```python
from build123d import *

# Parameters (mm, degrees)
SKETCH1_R               = 10
SKETCH1_R_2             = 4.425
BOSS_EXTRUDE1_DEPTH     = 2
SKETCH1_2_R             = 4.425
BOSS_EXTRUDE2_DEPTH     = 4.55
SKETCH2_R               = 2.75
SKETCH2_R_2             = 1.5
CUT_EXTRUDE1_DEPTH      = 3.5
CUT_EXTRUDE2_DEPTH      = 15.85605937
CUT_EXTRUDE2_DEPTH_BACK = 15.85605937
SKETCH2_3_R             = 1.5
SKETCH3_R               = 1.5
CUT_EXTRUDE3_DEPTH      = 15.370194849
CIRPATTERN1_COUNT       = 4
FILLET1_R               = 0.5


with BuildPart() as part:
    # Sketch1 → Boss-Extrude1 (new body)
    with BuildSketch(Plane(origin=(0, 0, 0), x_dir=(1, 0, 0), z_dir=(0, 1, 0))):
        with Locations(Location((0, 0, 0), (0, 0, 270))):
            Circle(SKETCH1_R)
        with Locations(Location((0, 0, 0), (0, 0, 270))):
            Circle(SKETCH1_R_2, mode=Mode.SUBTRACT)
    extrude(amount=BOSS_EXTRUDE1_DEPTH)

    # Sketch1_2 → Boss-Extrude2 (add)
    with BuildSketch(Plane(origin=(0, 0, 0), x_dir=(1, 0, 0), z_dir=(0, 1, 0))):
        with Locations(Location((0, 0, 0), (0, 0, 270))):
            Circle(SKETCH1_2_R)
    extrude(amount=BOSS_EXTRUDE2_DEPTH)

    # Sketch2 → Cut-Extrude1 (cut)
    # profile 1 of 2: a face of its own
    with BuildSketch(Plane(origin=(0, 4.55, 0), x_dir=(1, 0, 0), z_dir=(0, 1, 0))):
        with Locations(Location((0, 0, 0), (0, 0, 270))):
            Circle(SKETCH2_R)
        Circle(SKETCH2_R_2, mode=Mode.SUBTRACT)
    # profile 2 of 2: a face of its own
    with BuildSketch(Plane(origin=(0, 4.55, 0), x_dir=(1, 0, 0), z_dir=(0, 1, 0))):
        Circle(SKETCH2_R_2)
    extrude(amount=-CUT_EXTRUDE1_DEPTH, mode=Mode.SUBTRACT)

    # Sketch2_3 → Cut-Extrude2 (cut, two sides: drawn at the far end of the back side and taken through both)
    with BuildSketch(Plane(origin=(0, 4.55, 0), x_dir=(1, 0, 0), z_dir=(0, 1, 0)).offset(-CUT_EXTRUDE2_DEPTH_BACK)):
        with Locations(Location((0, 0, 0), (0, 0, 270))):
            Circle(SKETCH2_3_R)
    extrude(amount=CUT_EXTRUDE2_DEPTH + CUT_EXTRUDE2_DEPTH_BACK, mode=Mode.SUBTRACT)

    # Sketch3 → Cut-Extrude3 (cut, symmetric)
    with BuildSketch(Plane(origin=(0, 2, 0), x_dir=(1, 0, 0), z_dir=(0, 1, 0))):
        with Locations(Location((0, 7.2125, 0), (0, 0, 270))):
            Circle(SKETCH3_R)
    cut_extrude3 = extrude(amount=CUT_EXTRUDE3_DEPTH, both=True, mode=Mode.SUBTRACT)

    # CirPattern1: Cut-Extrude3 ×4 about axis
    cirpattern1_axis = Axis((0, 0, 0), (0, 1, 0))
    for i in range(1, CIRPATTERN1_COUNT):
        add(cut_extrude3.rotate(cirpattern1_axis, i * 360 / CIRPATTERN1_COUNT), mode=Mode.SUBTRACT)

    # Fillet1
    fillet1_edges = [part.edges().sort_by_distance(p)[0] for p in [
        (0, 4.55, -4.425),
        (0, 0, -10),
        (0, 2, -10),
    ]]
    fillet(fillet1_edges, radius=FILLET1_R)


solid = part.part
```
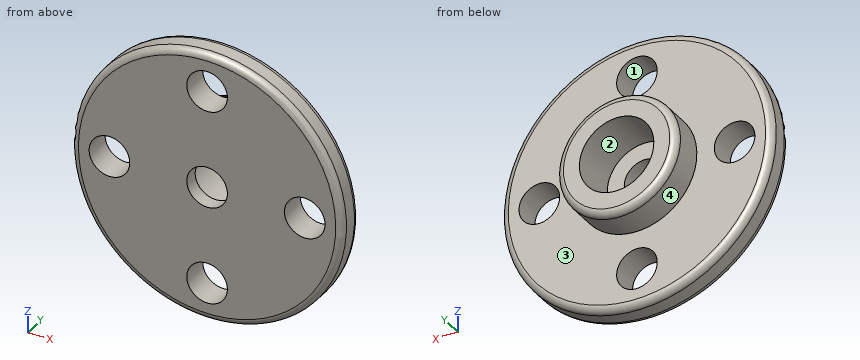
Verification items for the finished model (mm, model axes). Face numbers are marked on the shaded views. Coordinates: 2 decimals unless noted, no trailing zeros. Loops run counter-clockwise (first coordinate to the right, second up) from the corner with the lowest first, then second, coordinate; pieces in that order, holes last. Notation, with made-up numbers: (32, 21.5) -> (50, 21.5) arc R37 cw to (50, 58.5) -> close; hole circle Ø5 at (-3, 54.25). An arc over 180 degrees is marked (long way). Put each result on its own line as item: value.
1. Section check A-A, the plane z = 0. Give the number of separate pieces and of enclosed holes in the cut face, then the cut area to 3 significant figures.
Result set:
separate pieces: 4
enclosed holes: 0
area: 27.8 mm^2
2. Section check C-C, the plane y = 3.75. Record the boundary of the cut face in (x, z) (3 decimals).
Result set:
outline: circle Ø8.85 at (0, 0); hole circle Ø5.5 at (0, 0)
3. Thickness scan on line 1 (Z direction, x = -0.25, y = 1.15); line 2 (Z direction, x = -2, y = 4.05); line 3 (X direction, y = 2.9, z = -2.25). Record the ranges inside material, lowest first.
Result set:
line 1: z = -10 to -8.69, -5.73 to -2.74, 2.74 to 5.73, 8.69 to 10
line 2: z = -3.95 to -1.89, 1.89 to 3.95
line 3: x = -3.81 to -1.58, 1.58 to 3.81
4. Mould release check, pull along X, two halves, no side actions. Record for the marked faces 1, 2, 3 and 4: pulls with the +X half, pulls with the -X half, needs draft (parallel to the pull), parting line crosses it, or undercut.
Result set:
face 1: undercut
face 2: undercut
face 3: needs draft
face 4: parting line crosses it
5. Gauge pin test, flat ends, axial feed: P1, Ø5, axis at x = -7.21, z = 0, coming from the +Y side; P2, Ø2.5, axis at x = 0, z = -7.21, coming from the +Y side; P3, Ø1.5, axis at x = -1.5, y = 2, coming from the +Z side; P4, Ø5, axis at x = 0, z = 0, coming from the +Y side. Record the tip position at first contact, or that the pin passes through.
Result set:
P1: stops at y = 2
P2: passes through
P3: stops at z = 9.96
P4: stops at y = 1.05
